Geometry: final body of the model. Coordinates: model frame, mm. Face numbers are marked on the shaded views. A direction names the side the tool comes from. Coordinates: 2 decimals unless noted, no trailing zeros. Loops run counter-clockwise (first coordinate to the right, second up) from the corner with the lowest first, then second, coordinate; pieces in that order, holes last. Notation, with made-up numbers: (87.5, 75.25) - (143.5, 75.25) arc R9 cw to (143.5, 92.25) - close; hole circle Ø10 at (76, -17.75). An arc over 180 degrees is marked (long way). Put each result on its own line as item: value. Start each with the question number.
1) Contact query for flat-ended pins moving along their axis: pin 1 Ø1.5 at (x, z) = (39.5, 18.5) entering from -Y; pin 2 Ø1.5 at (y, z) = (16, 19.5) entering from +X; pin 3 Ø6.5 at (y, z) = (26.5, 21) entering from -X. Output: stop coordinate, or through.
2) Section D-D on x = 33.5. Output: boundary loops of the cut face in (y, z).
3) Section B-B on z = 7.5. Output: boundary loops of the cut face in (x, y).
4) Material intervals for line 1 along Y through (x, z) = (-40.5, 25); line 2 along Z through (x, y) = (38, -27); line 3 along X through (y, z) = (-27.5, 19), sorted ascending. Write a range as from..to.
5) Reachability of the marked faces 5, 6, 7 and 8 from +Z, -Z, +X, -X, +Y, -Y: full face, straight path, thin tool, end or side. Return the list, or none.
6) Section C-C on y = 11.5. Output: boundary loops of the cut face in (x, z), and give its area (3 significant figures).
7) Draft query along X for the marked faces 1, 2, 3 and 4. Return one class per face: +X half, -X half, draft (parallel to the pull), parting line (faces both ways), or undercut.
8) Section A-A on y = -17. Output: boundary loops of the cut face in (x, z), and give its area (3 significant figures).
```python
from build123d import *

# Parameters (mm, degrees)
F0_W     = 101.6
F0_H     = 63.5
F1_DEPTH = 10.16
F3_DEPTH = 30.48
F4_DEPTH = 25.4
F5_R     = 10.4245741623
F6_R     = 12.2642048969
F7_R     = 9.8113639175


with BuildPart() as f1:
    # F0 (on Top) → F1 (new body)
    with BuildSketch(Plane.XY):
        Rectangle(F0_W, F0_H)
    extrude(amount=F1_DEPTH)

    # F2 (on Top) → F3 (join)
    with BuildSketch(Plane.XY):
        with BuildLine():
            Line((-41.4277352393, 31.75), (-41.4277352393, 6.35))
            Line((-41.4277352393, 6.35), (-28.6113340408, 6.35))
            Line((-28.6113340408, 6.35), (-28.6113340408, -31.75))
            Line((-28.6113340408, -31.75), (-23.3824987947, -31.75))
            ThreePointArc((-23.3824987947, -31.75), (-16.5415723839, -15.1712032327), (0, -8.2407516258))
            ThreePointArc((0, -8.2407516258), (16.5415723839, -15.1712032327), (23.3824987947, -31.75))
            Line((23.3824987947, -31.75), (28.6113340408, -31.75))
            Line((28.6113340408, -31.75), (28.6113340408, 6.35))
            Line((28.6113340408, 6.35), (41.4277352393, 6.35))
            Line((41.4277352393, 6.35), (41.4277352393, 31.75))
            Line((41.4277352393, 31.75), (35.0195355713, 31.75))
            Line((35.0195355713, 31.75), (35.0195355713, 18.9336006641))
            Line((35.0195355713, 18.9336006641), (0, 18.9336006641))
            Line((0, 18.9336006641), (-35.0195355713, 18.9336006641))
            Line((-35.0195355713, 18.9336006641), (-35.0195355713, 31.75))
            Line((-35.0195355713, 31.75), (-41.4277352393, 31.75))
        make_face()
    extrude(amount=F3_DEPTH)

    # F4 (cut): a face of the model
    f4_faces = [f1.faces().sort_by_distance(p)[0] for p in [
        (0, -21.7845350745, 10.16),
    ]]
    extrude(f4_faces, amount=-F4_DEPTH, mode=Mode.SUBTRACT)

    # F5
    f5_edges = [f1.edges().sort_by_distance(p)[0] for p in [
        (50.8, -31.75, 5.08),
    ]]
    fillet(f5_edges, radius=F5_R)

    # F6
    f6_edges = [f1.edges().sort_by_distance(p)[0] for p in [
        (-50.8, -31.75, 5.08),
    ]]
    fillet(f6_edges, radius=F6_R)

    # F7
    f7_edges = [f1.edges().sort_by_distance(p)[0] for p in [
        (28.611334, 6.35, 20.32),
        (-28.611334, 6.35, 20.32),
    ]]
    fillet(f7_edges, radius=F7_R)


solid = f1.part
```
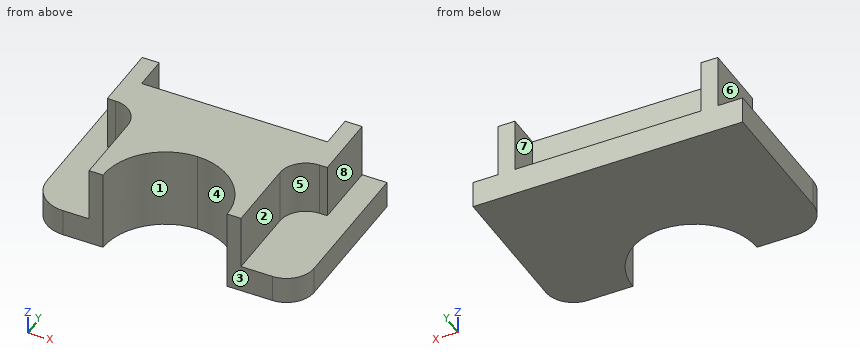
Answer block:
1. pin 1: stops at y = 6.35
1. pin 2: stops at x = 41.43
1. pin 3: stops at x = -41.43
2. outline: (-31.75, 0) - (31.75, 0) - (31.75, 10.16) - (18.93, 10.16) - (18.93, 30.48) - (5.03, 30.48) - (5.03, 10.16) - (-31.75, 10.16) - close
3. outline: (-50.8, -19.49) arc R12.26 ccw to (-38.54, -31.75) - (-23.38, -31.75) arc R23.51 cw to (0, -8.24) arc R23.51 cw to (23.38, -31.75) - (40.38, -31.75) arc R10.42 ccw to (50.8, -21.33) - (50.8, 31.75) - (-50.8, 31.75) - close
4. line 1: y = 6.35..31.75
4. line 2: z = 0..10.16
4. line 3: x = -28.61..-23, 23..28.61
5. face 5: +Z, +X, -Y
5. face 6: +Z, -X, +Y, -Y
5. face 7: +Z, +Y
5. face 8: +Z, +X, +Y, -Y
6. outline: (-50.8, 0) - (50.8, 0) - (50.8, 10.16) - (41.43, 10.16) - (41.43, 30.48) - (-41.43, 30.48) - (-41.43, 10.16) - (-50.8, 10.16) - close
6. area: 2,720 mm²
7. face 1: undercut
7. face 2: +X half
7. face 3: draft
7. face 4: undercut
8. outline: (-50.8, 0) - (-18.18, 0) - (-18.18, 30.48) - (-28.61, 30.48) - (-28.61, 10.16) - (-50.8, 10.16) - close; (18.18, 0) - (50.8, 0) - (50.8, 10.16) - (28.61, 10.16) - (28.61, 30.48) - (18.18, 30.48) - close
8. area: 1,090 mm²
